from build123d import *

# Parameters (mm, degrees)
CROQUIS1_W              = 4
CROQUIS1_H              = 4
SALIENTE_EXTRUIR1_DEPTH = 20
CROQUIS2_R              = 1.5
SALIENTE_EXTRUIR2_DEPTH = 3


with BuildPart() as part:
    # Croquis1 → Saliente-Extruir1 (new body)
    with BuildSketch(Plane.XY):
        Rectangle(CROQUIS1_W, CROQUIS1_H)
    extrude(amount=SALIENTE_EXTRUIR1_DEPTH)

    # Croquis2 → Saliente-Extruir2 (add)
    with BuildSketch(Plane(origin=(0, 0, 0), x_dir=(-1, 0, 0), z_dir=(0, 0, -1))):
        Circle(CROQUIS2_R)
    saliente_extruir2 = extrude(amount=SALIENTE_EXTRUIR2_DEPTH)

    # Simetría1: Saliente-Extruir2 across plane
    add(saliente_extruir2.mirror(Plane.XY.offset(10)))


solid = part.part
The listing builds one solid part. Answer for the finished solid, in the listing's coordinates (mm). A direction names the side the tool comes from. Coordinates: 2 decimals unless noted, no trailing zeros. Loops run counter-clockwise (first coordinate to the right, second up) from the corner with the lowest first, then second, coordinate; pieces in that order, holes last. Notation, with made-up numbers: (79.5, 74) -> (87.5, 74) arc R22 cw to (87.5, 95) -> close; hole circle Ø9 at (49, 65). An arc over 180 degrees is marked (long way). Write item = value, one per line. Start each with the question number.
1) A cutting plane is placed at A-A (x = 0). Give the vertices of the cut face in (y, z).
2) A cutting plane is placed at D-D (y = 1.75). Give the vertices of the cut face in (x, z), then the cut area to 3 significant figures.
3) Straight lines are drawn through the part: line 1 (Z direction, x = -1.3, y = 1.8); line 2 (X direction, y = -0.7, z = 22.25). For each, find the intervals that lie inside material, in ascending order. Write a range as from..to.
4) A tool of negligible diameter and unlimited length cuts with its end or side. For faces 1 (the face through (0.9, 1.4, 20)), 2 (the face through (0, 2, 10)), 3 (the face through (1.5, 0.07, -1.48)), from which of +Z, -Z, +X, -X, +Y, -Y can it reach the whole face along a straight path? Write none if from no direction.
5) A cutting plane is placed at C-C (z = -1). Give the vertices of the cut face in (x, y), then the cut area to 3 significant figures.
Responses:
q1.outline = (-2, 0) -> (-1.5, 0) -> (-1.5, -3) -> (1.5, -3) -> (1.5, 0) -> (2, 0) -> (2, 20) -> (1.5, 20) -> (1.5, 23) -> (-1.5, 23) -> (-1.5, 20) -> (-2, 20) -> close
q2.outline = (-2, 0) -> (2, 0) -> (2, 20) -> (-2, 20) -> close
q2.area = 80.0 mm²
q3.line_1 = 0..20
q3.line_2 = -1.33..1.33
q4.face_1 = +Z
q4.face_2 = +Z, -Z, +X, -X, +Y
q4.face_3 = -Z
q5.outline = circle Ø3 at (0, 0)
q5.area = 7.07 mm²
